For this review, use the dimensioned drawing (mm, ordinates from the lowest corner) and the shaded views. A direction names the side the tool comes from. Give positions to 0.01 mm unless a question says otherwise; leave off trailing zeros. Write each loop counter-clockwise with the first axis right and the second up, starting at its lowest first coordinate (ties: lowest second). Pieces come first, ordered by that corner, then holes. Notation, with made-up numbers: (29.5, 81) -> (80.5, 81) arc R28 cw to (80.5, 114) -> close; hole circle Ø10 at (2.25, 13). An arc over 180 degrees is marked (long way). Return JSON: item names as keys, results as strings.
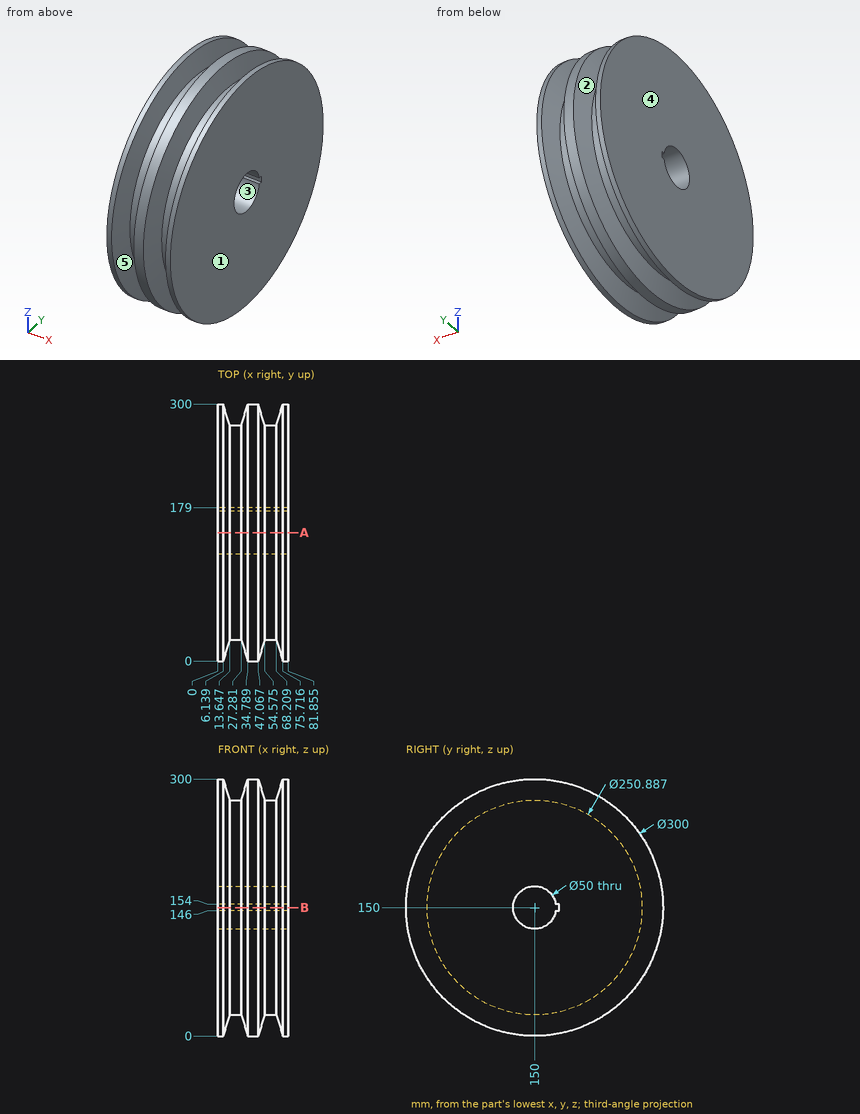
1. For pin 1 (1.5 mm diameter, centred on y = 53, z = 203, fed in from -X); pin 2 (1 mm diameter, centred on x = 60, z = 176, fed in from -Y) (1 decimal); pin 3 (5 mm diameter, centred on x = 49.5, y = 178, fed in from +Z); pin 4 (10 mm diameter, centred on x = 46, y = 136.5, fed in from -Z), all flat-tipped, find the tip position at first contact; note any pin that passes through.
Results found:
{"pin 1": "stops at x = 0", "pin 2": "stops at y = 27.2", "pin 3": "stops at z = 297.47", "pin 4": "stops at z = 0.24"}
2. The part is to be moulded in two halves that separate along X. For the marked faces 3, 4 and 5, say which applies: +X half, -X half, draft (parallel to the pull), parting line (faces both ways), or undercut.
Results found:
{"face 3": "draft", "face 4": "-X half", "face 5": "undercut"}
3. Add section B-B, the plane z = 150. State the section outline as (x, y) points (1 decimal), plus the area to 3 significant figures.
Results found:
{"outline": "(0, 0) -> (6.1, 0) -> (13.6, 24.6) -> (27.3, 24.6) -> (34.8, 0) -> (47.1, 0) -> (54.6, 24.6) -> (68.2, 24.6) -> (75.7, 0) -> (81.9, 0) -> (81.9, 125) -> (0, 125) -> close; (0, 179) -> (81.9, 179) -> (81.9, 300) -> (75.7, 300) -> (68.2, 275.4) -> (54.6, 275.4) -> (47.1, 300) -> (34.8, 300) -> (27.3, 275.4) -> (13.6, 275.4) -> (6.1, 300) -> (0, 300) -> close", "area": "18,100 mm²"}
4. For the marked faces 1 and 2, list the 3-axis set-ups (+Z, -Z, +X, -X, +Y, -Y) from which the entire face can be reached by the end or side of a thin tool; tool diameter is ignored.
Results found:
{"face 1": "+Z, -Z, +X, +Y, -Y", "face 2": "none"}
5. Add section A-A, the plane y = 150. State the section outline as (x, z) points (1 decimal), plus the area to 3 significant figures.
Results found:
{"outline": "(0, 0) -> (6.1, 0) -> (13.6, 24.6) -> (27.3, 24.6) -> (34.8, 0) -> (47.1, 0) -> (54.6, 24.6) -> (68.2, 24.6) -> (75.7, 0) -> (81.9, 0) -> (81.9, 125) -> (0, 125) -> close; (0, 175) -> (81.9, 175) -> (81.9, 300) -> (75.7, 300) -> (68.2, 275.4) -> (54.6, 275.4) -> (47.1, 300) -> (34.8, 300) -> (27.3, 275.4) -> (13.6, 275.4) -> (6.1, 300) -> (0, 300) -> close", "area": "18,400 mm²"}
6. To check wall thickness, follow probe 1 along Y at (x, z) = (64, 150); probe 2 along X at (y, z) = (18, 156.5) (1 decimal); probe 3 along Z at (x, y) = (63, 148). State the ranges of each line that lie inside material, in increasing order.
Results found:
{"probe 1": "y = 24.56 to 125, 179 to 275.44", "probe 2": "x = 0 to 11.6, 29.3 to 52.5, 70.3 to 81.9", "probe 3": "z = 24.57 to 125.08, 174.92 to 275.43"}
